Part model, mm, in its own coordinate system. Coordinates: 2 decimals unless noted, no trailing zeros. Write each loop counter-clockwise with the first axis right and the second up, starting at its lowest first coordinate (ties: lowest second). Pieces come first, ordered by that corner, then holes. Notation, with made-up numbers: M 21,51.25 L 47,51.25 A25 cw 47,87.25 Z; hole C 85.25,40.5 d6. An arc over 180 degrees is marked long. Use a Markdown table: item, result. Add a question column.
Q1. Wall check: L1, parallel to Z at x = 0, y = -1.2; L2, parallel to X at y = -1.1, z = -13; L3, parallel to Z at x = -0.25, y = -0.2. Give the ranges that are in metal, low to high. Write a range as from..to.
Q2. Slice it at C-C on y = -2.6. Write the cut outline in (x, z), then the cut area to 3 significant figures.
Q3. Mould opens along Z. For faces 1 (the flat face through (0, 0, 0)), 2 (the cylindrical face through (-1.183, -1.521, -14.855)), 3 (the cylindrical face through (-1.183, -1.521, 11.145)), 4 (the cylindrical face through (-0.028, -2.715, 19.699)) say: released by +Z, released by -Z, zero draft, split by the parting line, or undercut.
Q4. Slice it at D-D on z = 8.5. Write the cut outline in (x, y), then the cut area to 3 significant figures.
Q5. Slice it at B-B on z = -13. Write the cut outline in (x, y), then the cut area to 3 significant figures.
Q6. Slice it at A-A on x = 0. Write the cut outline in (y, z), then the cut area to 3 significant figures.
from build123d import *

# Parameters (mm, degrees)
F0_W           = 12
F0_H           = 40
F1_DEPTH       = 3
F2_R           = 4
F3_R           = 1
F5_D           = 4.4
F5_DEPTH       = 30
F5_CBORE_D     = 4.4
F5_CBORE_DEPTH = 4


with BuildPart() as f1:
    # F0 (on Front) → F1 (new body)
    with BuildSketch(Plane.XZ):
        Rectangle(F0_W, F0_H)
    extrude(amount=F1_DEPTH)

    # F2
    f2_edges = [f1.edges().sort_by_distance(p)[0] for p in [
        (6, -1.5, 20),
        (-6, -1.5, 20),
        (6, -1.5, -20),
        (-6, -1.5, -20),
    ]]
    fillet(f2_edges, radius=F2_R)

    # F3
    f3_edges = [f1.edges().sort_by_distance(p)[0] for p in [
        (6, -3, 0),
        (6, 0, 0),
        (-6, 0, 0),
        (-6, -3, 0),
    ]]
    fillet(f3_edges, radius=F3_R)

    # F5
    with Locations(Plane(origin=(0, 0, 0), x_dir=(1, 0, 0), z_dir=(0, 1, 0))):
        with Locations((0, 13), (0, -13)):
            CounterBoreHole(F5_D / 2, F5_CBORE_D / 2, F5_CBORE_DEPTH, depth=F5_DEPTH)


solid = f1.part
Recorded:
| question | item | result |
|---|---|---|
| 1 | L1 | -20..-15.2, -10.8..10.8, 15.2..20 |
| 1 | L2 | -6..-2.2, 2.2..6 |
| 1 | L3 | -19.6..-15.19, -10.81..10.81, 15.19..19.6 |
| 2 | outline | M -5.8,-16 A3.8 ccw -2,-19.8 L 2,-19.8 A3.8 ccw 5.8,-16 L 5.8,16 A3.8 ccw 2,19.8 L -2,19.8 A3.8 ccw -5.8,16 Z; hole C 0,-13 d4.4; hole C 0,13 d4.4 |
| 2 | area | 417 mm² |
| 3 | face 1 | zero draft |
| 3 | face 2 | undercut |
| 3 | face 3 | undercut |
| 3 | face 4 | released by +Z |
| 4 | outline | M -6,-2 A1 ccw -5,-3 L 5,-3 A1 ccw 6,-2 L 6,-1 A1 ccw 5,0 L -5,0 A1 ccw -6,-1 Z |
| 4 | area | 35.1 mm² |
| 5 | outline | M -6,-2 A1 ccw -5,-3 L -2.2,-3 L -2.2,0 L -5,0 A1 ccw -6,-1 Z; M 2.2,-3 L 5,-3 A1 ccw 6,-2 L 6,-1 A1 ccw 5,0 L 2.2,0 Z |
| 5 | area | 21.9 mm² |
| 6 | outline | M -3,-19 A1 ccw -2,-20 L -1,-20 A1 ccw 0,-19 L 0,-15.2 L -3,-15.2 Z; M -3,-10.8 L 0,-10.8 L 0,10.8 L -3,10.8 Z; M -3,15.2 L 0,15.2 L 0,19 A1 ccw -1,20 L -2,20 A1 ccw -3,19 Z |
| 6 | area | 92.7 mm² |
